Input: part model. Units: mm. Frame: model coordinates. Give positions to 0.01 mm unless a question says otherwise; leave off trailing zeros. Order: outer loops, then holes, each group sorted by start corner. A loop starts at its lowest first (then second) coordinate and runs counter-clockwise, first axis right, second up. Notation, with made-up numbers: (7, 44) - (59, 44) arc R19 cw to (59, 59) - close; hole circle Ø10 at (35, 5). An arc over 180 degrees is marked (long way). Use a Markdown table: item, result.
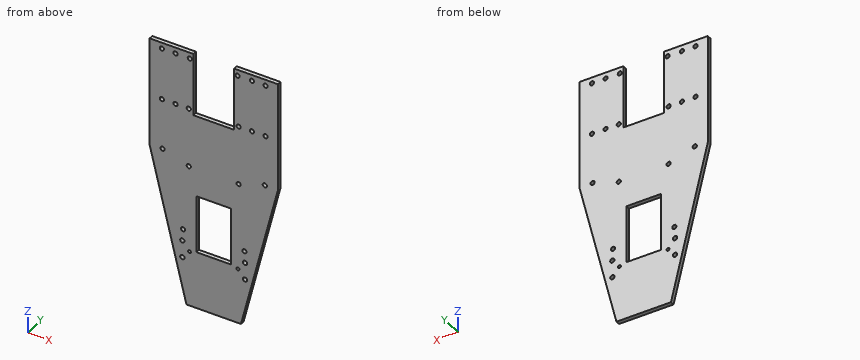
from build123d import *

# Parameters (mm, degrees)
BODY_DEPTH             = 3
SKETCH4_R              = 1.55
MOTOR_MOUNT_DEPTH      = 3
SKETCH5_R              = 1.1
SKETCH5_W              = 25.4
SKETCH5_H              = 42
PROTOBOARD_MOUNT_DEPTH = 10
SKETCH6_R              = 1.6
CASTER_MOUNT_DEPTH     = 10
SKETCH8_R              = 1.55
STAND_OFF_MOUNT_DEPTH  = 10


with BuildPart() as part:
    # Sketch3 → Body (new body)
    with BuildSketch(Plane(origin=(0, 0, 0), x_dir=(1, 0, 0), z_dir=(0, 1, 0))):
        Polygon((-15, -46), (-47, -46), (-47, 34), (-20, 144), (20, 144), (47, 34), (47, -46), (15, -46), (15, 0), (-15, 0), align=None)
    extrude(amount=BODY_DEPTH)

    # Sketch4 → Motor Mount (cut)
    with BuildSketch(Plane(origin=(0, 3, 0), x_dir=(1, 0, 0), z_dir=(0, 1, 0))):
        with Locations(Location((-38, -3.65, 0), (0, 0, 270))):
            Circle(SKETCH4_R)
        with Locations(Location((-28, -3.65, 0), (0, 0, 270))):
            Circle(SKETCH4_R)
        with Locations(Location((-38, -41.6, 0), (0, 0, 270))):
            Circle(SKETCH4_R)
        with Locations(Location((-28, -41.6, 0), (0, 0, 270))):
            Circle(SKETCH4_R)
        with Locations(Location((-18.29, -3.65, 0), (0, 0, 270))):
            Circle(SKETCH4_R)
        with Locations(Location((18.29, -3.65, 0), (0, 0, 90))):
            Circle(SKETCH4_R)
        with Locations(Location((28, -41.6, 0), (0, 0, 90))):
            Circle(SKETCH4_R)
        with Locations(Location((38, -41.6, 0), (0, 0, 90))):
            Circle(SKETCH4_R)
        with Locations(Location((28, -3.65, 0), (0, 0, 90))):
            Circle(SKETCH4_R)
        with Locations(Location((38, -3.65, 0), (0, 0, 90))):
            Circle(SKETCH4_R)
        with Locations(Location((-18.29, 39.53, 0), (0, 0, 270))):
            Circle(SKETCH4_R)
        with Locations(Location((18.29, 39.53, 0), (0, 0, 270))):
            Circle(SKETCH4_R)
    extrude(amount=-MOTOR_MOUNT_DEPTH, mode=Mode.SUBTRACT)

    # Sketch5 → Protoboard Mount (cut)
    with BuildSketch(Plane(origin=(0, 3, 0), x_dir=(1, 0, 0), z_dir=(0, 1, 0))):
        with Locations(Location((-17.8, 103.5, 0), (0, 0, 270))):
            Circle(SKETCH5_R)
        with Locations(Location((17.8, 103.5, 0), (0, 0, 270))):
            Circle(SKETCH5_R)
        with Locations((0, 81)):
            Rectangle(SKETCH5_W, SKETCH5_H)
    extrude(amount=-PROTOBOARD_MOUNT_DEPTH, mode=Mode.SUBTRACT)

    # Sketch6 → Caster Mount (cut)
    with BuildSketch(Plane(origin=(0, 3, 0), x_dir=(1, 0, 0), z_dir=(0, 1, 0))):
        with Locations(Location((-23, 109.5, 0), (0, 0, 270))):
            Circle(SKETCH6_R)
        with Locations(Location((-23, 97, 0), (0, 0, 270))):
            Circle(SKETCH6_R)
        with Locations(Location((23, 97, 0), (0, 0, 270))):
            Circle(SKETCH6_R)
        with Locations(Location((23, 109.5, 0), (0, 0, 270))):
            Circle(SKETCH6_R)
    extrude(amount=-CASTER_MOUNT_DEPTH, mode=Mode.SUBTRACT)

    # Sketch8 → Stand Off Mount (cut)
    with BuildSketch(Plane(origin=(0, 3, 0), x_dir=(1, 0, 0), z_dir=(0, 1, 0))):
        with Locations(Location((-22.5, 88.4, 0), (0, 0, 270))):
            Circle(SKETCH8_R)
        with Locations(Location((22.5, 88.4, 0), (0, 0, 270))):
            Circle(SKETCH8_R)
        with Locations(Location((37.5, 33.4, 0), (0, 0, 270))):
            Circle(SKETCH8_R)
        with Locations(Location((-37.5, 33.4, 0), (0, 0, 270))):
            Circle(SKETCH8_R)
        with Locations(Location((-17.5, -41.6, 0), (0, 0, 270))):
            Circle(SKETCH8_R)
        with Locations(Location((17.5, -41.6, 0), (0, 0, 270))):
            Circle(SKETCH8_R)
    extrude(amount=-STAND_OFF_MOUNT_DEPTH, mode=Mode.SUBTRACT)


solid = part.part
1. Section query C-C (y = 1.2). State how many separate pieces and enclosed holes the cut face has, then the cut area to 3 significant figures.
Response:
| item | result |
|---|---|
| separate pieces | 1 |
| enclosed holes | 25 |
| area | 12,300 mm^2 |
2. Material intervals for line 1 along Z through (x, y) = (-2, 0.4); line 2 along Z through (x, y) = (-18, 0.85); line 3 along X through (y, z) = (1.6, 5.5), sorted ascending.
Response:
| item | result |
|---|---|
| line 1 | z = -144 to -102, -60 to 0 |
| line 2 | z = -144 to -104.58, -102.42 to -41.05, -38.01 to 2.13, 5.17 to 40.13, 43.07 to 46 |
| line 3 | x = -47 to -15, 15 to 47 |
3. Section query D-D (z = -125). Return loops of the section in (x, y), then the cut area to 3 significant figures.
Response:
| item | result |
|---|---|
| outline | (-24.66, 0) - (24.66, 0) - (24.66, 3) - (-24.66, 3) - close |
| area | 148 mm^2 |
4. Section query A-A (x = -4). Return loops of the section in (y, z), then the cut area to 3 significant figures.
Response:
| item | result |
|---|---|
| outline | (0, -144) - (3, -144) - (3, -102) - (0, -102) - close; (0, -60) - (3, -60) - (3, 0) - (0, 0) - close |
| area | 306 mm^2 |
5. Section query B-B (z = -76). Return loops of the section in (x, y).
Response:
| item | result |
|---|---|
| outline | (-36.69, 0) - (-12.7, 0) - (-12.7, 3) - (-36.69, 3) - close; (12.7, 0) - (36.69, 0) - (36.69, 3) - (12.7, 3) - close |
6. Pin query (flat end, axial travel): pin 1 (3 mm diameter, centred on x = -38, z = 41.6, fed in from +Y); pin 2 (4 mm diameter, centred on x = 37.5, z = -33.4, fed in from -Y); pin 3 (1.5 mm diameter, centred on y = 1.5, z = -85.5, fed in from -X); pin 4 (1.5 mm diameter, centred on x = -2, y = 1.5, fed in from +Z). Return the tip coordinate at first contact, or that it passes through.
Response:
| item | result |
|---|---|
| pin 1 | passes through |
| pin 2 | stops at y = 0 |
| pin 3 | stops at x = -34.54 |
| pin 4 | stops at z = 0 |
